```python
from build123d import *

# Parameters (mm, degrees)
BOSS_EXTRUDE1_DEPTH          = 4
SKETCH2_W                    = 4
SKETCH2_H                    = 32
BOSS_EXTRUDE2_DEPTH          = 72
CUT_EXTRUDE1_DEPTH           = 109.664621658
SKETCH4_W                    = 12.6
SKETCH4_H                    = 4
SKETCH4_W_2                  = 12.599860781
BOSS_EXTRUDE3_DEPTH          = 4
SKETCH5_R                    = 1
CUT_EXTRUDE2_DEPTH           = 4
CUT_EXTRUDE2_DRAFT           = -1
CUT_EXTRUDE2_PROFILE_2_DEPTH = 4
CUT_EXTRUDE2_PROFILE_2_DRAFT = -1
CUT_EXTRUDE4_DEPTH           = 102.980390272
BOSS_EXTRUDE6_DEPTH          = 32
BOSS_EXTRUDE7_DEPTH          = 2
SKETCH14_R                   = 18
SKETCH14_R_2                 = 16
BOSS_EXTRUDE8_DEPTH          = 4
SKETCH15_R                   = 2
CUT_EXTRUDE5_DEPTH           = 4
SKETCH16_R                   = 4
SKETCH16_R_2                 = 2
CUT_EXTRUDE6_DEPTH           = 2
SKETCH17_W                   = 5
SKETCH17_H                   = 10
CUT_EXTRUDE7_DEPTH           = 10
BOSS_EXTRUDE9_DEPTH          = 2
MIRROR6_COPY_1_DEPTH         = 2
FILLET1_R                    = 10
FILLET2_R                    = 10


with BuildPart() as part:
    # Sketch1 → Boss-Extrude1 (new body)
    with BuildSketch(Plane(origin=(0, 0, 0), x_dir=(1, 0, 0), z_dir=(0, 1, 0))):
        with BuildLine():
            Line((0, 16), (60, 16))
            Line((60, 16), (60, -16))
            Line((60, -16), (0, -16))
            ThreePointArc((0, -16), (-16, 0), (0, 16))
        make_face()
    boss_extrude1 = extrude(amount=BOSS_EXTRUDE1_DEPTH)

    # Sketch2 → Boss-Extrude2 (add)
    with BuildSketch(Plane(origin=(0, 4, 0), x_dir=(1, 0, 0), z_dir=(0, 1, 0))):
        with Locations((58, 0)):
            Rectangle(SKETCH2_W, SKETCH2_H)
    extrude(amount=BOSS_EXTRUDE2_DEPTH)

    # Mirror1: Boss-Extrude1 across plane
    add(boss_extrude1.mirror(Plane(origin=(0, 38, 0), x_dir=(0, 0, 1), z_dir=(0, -1, 0))))

    # Sketch3 → Cut-Extrude1 (cut, through all)
    with BuildSketch(Plane(origin=(60, 0, 0), x_dir=(0, 0, -1), z_dir=(1, 0, 0))):
        with BuildLine():
            ThreePointArc((-2.594812436, 43.59757706), (0, 31.830241454), (2.594812436, 43.59757706))
            ThreePointArc((2.594812436, 43.59757706), (0, 46.625832401), (-2.594812436, 43.59757706))
        make_face()
    extrude(amount=-CUT_EXTRUDE1_DEPTH, mode=Mode.SUBTRACT)

    # Sketch4 → Boss-Extrude3 (add)
    with BuildSketch(Plane.ZY.offset(-56)):
        with Locations((0, 57.55)):
            Rectangle(SKETCH4_W, SKETCH4_H)
        with Locations((8.8752e-05, 29.45)):
            Rectangle(SKETCH4_W_2, SKETCH4_H)
    extrude(amount=BOSS_EXTRUDE3_DEPTH)


with BuildPart() as cut_extrude2_tool:
    # Sketch5 → Cut-Extrude2 (with draft: the straight prism first)
    with BuildSketch(Plane.ZY.offset(-52)):
        with Locations((0, 57.275)):
            Circle(SKETCH5_R)
    extrude(amount=-CUT_EXTRUDE2_DEPTH)
    # Cut-Extrude2: the draft: its side faces are tilted about the plane it starts from
    cut_extrude2_sides = [cut_extrude2_tool.faces().sort_by_distance(p)[0] for p in [
        (54, 57.275, -1),
    ]]
    draft(cut_extrude2_sides, Plane.ZY.offset(-52), CUT_EXTRUDE2_DRAFT)


with BuildPart() as part_1:
    add(part.part)

    # Cut-Extrude2: cut by cut_extrude2_tool
    add(cut_extrude2_tool.part, mode=Mode.SUBTRACT)


with BuildPart() as cut_extrude2_profile_2_tool:
    # Sketch5 → Cut-Extrude2 profile 2 (with draft: the straight prism first)
    with BuildSketch(Plane.ZY.offset(-52)):
        with Locations((0.01512814, 29.732868428)):
            Circle(SKETCH5_R)
    extrude(amount=-CUT_EXTRUDE2_PROFILE_2_DEPTH)
    # Cut-Extrude2 profile 2: the draft: its side faces are tilted about the plane it starts from
    cut_extrude2_profile_2_sides = [cut_extrude2_profile_2_tool.faces().sort_by_distance(p)[0] for p in [
        (54, 29.732868428, -0.98487186),
    ]]
    draft(cut_extrude2_profile_2_sides, Plane.ZY.offset(-52), CUT_EXTRUDE2_PROFILE_2_DRAFT)


with BuildPart() as part_2:
    add(part_1.part)

    # Cut-Extrude2 profile 2: cut by cut_extrude2_profile_2_tool
    add(cut_extrude2_profile_2_tool.part, mode=Mode.SUBTRACT)

    # Sketch11 → Cut-Extrude4 (cut, through all)
    with BuildSketch(Plane.XY.offset(16)):
        Polygon((56, 59.55), (30, 72), (30, 76), (60, 76), (60, 59.55), align=None)
        Polygon((60, 0), (60, 14.79), (56, 14.79), (30, 4), (30, 0), align=None)
    extrude(amount=-CUT_EXTRUDE4_DEPTH, mode=Mode.SUBTRACT)


with BuildPart() as cut_extrude4_piece_1:
    # of the separate pieces the step leaves, piece 1, a body of its own (cut_extrude4_pieces)
    add(part_2.part.solids().sort_by_distance((60, 59.55, -16))[0])



with BuildPart() as cut_extrude4_piece_2:
    # of the separate pieces the step leaves, piece 2, a body of its own (cut_extrude4_pieces)
    add(part_2.part.solids().sort_by_distance((0, 0, -16))[0])


with BuildPart() as cut_extrude4_piece_3:
    # of the separate pieces the step leaves, piece 3, a body of its own (cut_extrude4_pieces)
    add(part_2.part.solids().sort_by_distance((0, 76, -16))[0])


with BuildPart() as cut_extrude4_piece_1_1:
    add(cut_extrude4_piece_1.part)

    add(cut_extrude4_piece_2.part)  # Boss-Extrude6 merges Cut-Extrude4 piece 2

    add(cut_extrude4_piece_3.part)  # Boss-Extrude6 merges Cut-Extrude4 piece 3
    # Sketch12 → Boss-Extrude6 (add, through all)
    with BuildSketch(Plane.XY.offset(16)):
        Polygon((30, 72), (56, 59.55), (60, 59.55), (60, 62.55), (30, 76), align=None)
        Polygon((30, 4), (56, 14.79), (60, 14.79), (60, 11.79), (30, 0), align=None)
    extrude(amount=-BOSS_EXTRUDE6_DEPTH)

    # Sketch13 → Boss-Extrude7 (add)
    with BuildSketch(Plane.XY.offset(16)):
        Polygon((30, 76), (30, 0), (60, 11.79), (60, 62.55), align=None)
    boss_extrude7 = extrude(amount=-BOSS_EXTRUDE7_DEPTH)

    # Mirror2: Boss-Extrude7 across plane
    add(boss_extrude7.mirror(Plane.XY))

    # Sketch14 → Boss-Extrude8 (add)
    with BuildSketch(Plane(origin=(0, 76, 0), x_dir=(1, 0, 0), z_dir=(0, 1, 0))):
        Circle(SKETCH14_R)
        Circle(SKETCH14_R_2, mode=Mode.SUBTRACT)
    boss_extrude8 = extrude(amount=-BOSS_EXTRUDE8_DEPTH)

    # Sketch15 → Cut-Extrude5 (cut)
    with BuildSketch(Plane(origin=(0, 76, 0), x_dir=(1, 0, 0), z_dir=(0, 1, 0))):
        with Locations(Location((-13.5, 0, 0), (0, 0, 270))):
            Circle(SKETCH15_R)
        with Locations(Location((-4.171729424, 12.83926297, 0), (0, 0, 270))):
            Circle(SKETCH15_R)
        with Locations(Location((10.921729424, 7.935100906, 0), (0, 0, 270))):
            Circle(SKETCH15_R)
        with Locations(Location((10.921729424, -7.935100906, 0), (0, 0, 270))):
            Circle(SKETCH15_R)
        with Locations(Location((-4.171729424, -12.83926297, 0), (0, 0, 270))):
            Circle(SKETCH15_R)
    cut_extrude5 = extrude(amount=-CUT_EXTRUDE5_DEPTH, mode=Mode.SUBTRACT)

    # Mirror3: Boss-Extrude8, Cut-Extrude5 across plane
    add(boss_extrude8.mirror(Plane(origin=(0, 38, 0), x_dir=(0, 0, 1), z_dir=(0, -1, 0))))
    add(cut_extrude5.mirror(Plane(origin=(0, 38, 0), x_dir=(0, 0, 1), z_dir=(0, -1, 0))), mode=Mode.SUBTRACT)

    # Sketch16 → Cut-Extrude6 (cut)
    # profile 1 of 5: a face of its own
    with BuildSketch(Plane.XZ):
        with Locations(Location((-4.171729424, 12.83926297, 0), (0, 0, 270))):
            Circle(SKETCH16_R)
        with Locations(Location((-4.171729424, 12.83926297, 0), (0, 0, 270))):
            Circle(SKETCH16_R_2, mode=Mode.SUBTRACT)
    # profile 2 of 5: a face of its own
    with BuildSketch(Plane.XZ):
        with Locations(Location((10.921729424, 7.935100906, 0), (0, 0, 270))):
            Circle(SKETCH16_R)
        with Locations(Location((10.921729424, 7.935100906, 0), (0, 0, 270))):
            Circle(SKETCH16_R_2, mode=Mode.SUBTRACT)
    # profile 3 of 5: a face of its own
    with BuildSketch(Plane.XZ):
        with Locations(Location((10.921729424, -7.935100906, 0), (0, 0, 270))):
            Circle(SKETCH16_R)
        with Locations(Location((10.921729424, -7.935100906, 0), (0, 0, 270))):
            Circle(SKETCH16_R_2, mode=Mode.SUBTRACT)
    # profile 4 of 5: a face of its own
    with BuildSketch(Plane.XZ):
        with Locations(Location((-4.171729424, -12.83926297, 0), (0, 0, 270))):
            Circle(SKETCH16_R)
        with Locations(Location((-4.171729424, -12.83926297, 0), (0, 0, 270))):
            Circle(SKETCH16_R_2, mode=Mode.SUBTRACT)
    # profile 5 of 5: a face of its own
    with BuildSketch(Plane.XZ):
        with Locations(Location((-13.5, 0, 0), (0, 0, 270))):
            Circle(SKETCH16_R)
        with Locations(Location((-13.5, 0, 0), (0, 0, 270))):
            Circle(SKETCH16_R_2, mode=Mode.SUBTRACT)
    cut_extrude6 = extrude(amount=-CUT_EXTRUDE6_DEPTH, mode=Mode.SUBTRACT)

    # Mirror4: Cut-Extrude6 across plane
    add(cut_extrude6.mirror(Plane(origin=(0, 38, 0), x_dir=(0, 0, 1), z_dir=(0, -1, 0))), mode=Mode.SUBTRACT)

    # Sketch17 → Cut-Extrude7 (cut)
    with BuildSketch(Plane(origin=(0, 0, -16), x_dir=(-1, 0, 0), z_dir=(0, 0, -1))):
        with Locations((-45, 38)):
            Rectangle(SKETCH17_W, SKETCH17_H)
    extrude(amount=-CUT_EXTRUDE7_DEPTH, mode=Mode.SUBTRACT)

    # Sketch18 → Boss-Extrude9 (add)
    with BuildSketch(Plane(origin=(0, 0, -16), x_dir=(-1, 0, 0), z_dir=(0, 0, -1))):
        Polygon((-30, 11), (-27, 8), (-26, 7), (-23, 4), (-30, 4), align=None)
    boss_extrude9 = extrude(amount=-BOSS_EXTRUDE9_DEPTH)

    # Mirror5: Boss-Extrude9 across plane
    add(boss_extrude9.mirror(Plane.XY))

    # Mirror6: Boss-Extrude9 across plane
    add(boss_extrude9.mirror(Plane(origin=(0, 38, 0), x_dir=(0, 0, 1), z_dir=(0, -1, 0))))

    # Mirror6 copy 1 sketch → Mirror6 copy 1 (add)
    with BuildSketch(Plane(origin=(0, 76, 16), x_dir=(-1, 0, 0), z_dir=(0, 0, 1))):
        Polygon((-30, 11), (-27, 8), (-26, 7), (-23, 4), (-30, 4), align=None)
    extrude(amount=-MIRROR6_COPY_1_DEPTH)

    # Fillet1
    fillet1_edges = [cut_extrude4_piece_1_1.edges().sort_by_distance(p)[0] for p in [
        (30, 72, 0),
    ]]
    fillet(fillet1_edges, radius=FILLET1_R)

    # Fillet2
    fillet2_edges = [cut_extrude4_piece_1_1.edges().sort_by_distance(p)[0] for p in [
        (30, 4, 0),
    ]]
    fillet(fillet2_edges, radius=FILLET2_R)


solid = cut_extrude4_piece_1_1.part
```
Check sheet for the modelled part. Datum: model origin and axes. Units: mm. A direction names the side the tool comes from. Round coordinates to 2 decimals unless told otherwise and drop trailing zeros. Loops run counter-clockwise (first coordinate to the right, second up) from the corner with the lowest first, then second, coordinate; pieces in that order, holes last. Notation, with made-up numbers: M -8,-22.75 L 29,-22.75 A27 cw 29,0.25 Z; hole C -39,-13.75 d3. An arc over 180 degrees is marked long. Answer as a JSON object with one key per item and string values.
1. Section check D-D (y = 20). Record the boundary of the cut face in (x, z), plus the area to 3 significant figures.
Reply:
{"outline": "M 30,-16 L 60,-16 L 60,16 L 30,16 L 30,14 L 56,14 L 56,-14 L 30,-14 Z", "area": "232 mm²"}
2. Access from +Z, -Z, +X, -X, +Y, -Y to the whole of each face (thin tool, end or side, straight path). Record for faces 1 (the flat face through (45, 33, -15)), 2 (the flat face through (26, 69, -15)), 3 (the cylindrical face through (13.63, 75.01, 10.88)).
Reply:
{"face 1": "-Z", "face 2": "+Z, -Z, -X", "face 3": "+Y"}
3. Section check C-C (x = 1). Record the boundary of the cut face in (y, z), plus the area to 3 significant figures.
Reply:
{"outline": "M 0,-17.97 L 4,-17.97 L 4,17.97 L 0,17.97 Z; M 72,-17.97 L 76,-17.97 L 76,17.97 L 72,17.97 Z", "area": "288 mm²"}
4. Section check B-B (z = 13). State how many separate pieces and enclosed holes the cut face has, plus the area to 3 significant figures.
Reply:
{"separate pieces": "3", "enclosed holes": "0", "area": "728 mm²"}
5. Mould release check, pull along X, two halves, no side actions. Record for faces 4 (the flat face through (5, 4, 0)), 5 (the flat face through (30, 38, 15)), 6 (the flat face through (13, 2, -9)): pulls with the +X half, pulls with the -X half, needs draft (parallel to the pull), parting line crosses it, or undercut.
Reply:
{"face 4": "needs draft", "face 5": "pulls with the -X half", "face 6": "undercut"}
6. Gauge pin test, flat ends, axial feed: P1, Ø12, axis at y = 11.5, z = -2.5, coming from the -X side; P2, Ø4, axis at y = 61, z = -6.5, coming from the -X side; P3, Ø7, axis at x = -4.17, z = -12.84, coming from the +Y side. Record the tip position at first contact, or that the pin passes through.
Reply:
{"P1": "stops at x = 33.61", "P2": "stops at x = 48.8", "P3": "stops at y = 74"}
7. Scan lines: line 1 (Y direction, x = 17, z = 9); line 2 (Z direction, x = 41, y = 44); line 3 (Y direction, x = 7, z = -8). Record each from-to range of solid material in increasing order.
Reply:
{"line 1": "y = 0 to 4, 72 to 76", "line 2": "z = -16 to -14, 14 to 16", "line 3": "y = 2 to 4, 72 to 74"}
8. Section check A-A (y = 38). Record the boundary of the cut face in (x, z), plus the area to 3 significant figures.
Reply:
{"outline": "M 30,-16 L 42.5,-16 L 42.5,-14 L 30,-14 Z; M 30,14 L 56,14 L 56,6.17 L 60,6.17 L 60,16 L 30,16 Z; M 47.5,-16 L 60,-16 L 60,-6.17 L 56,-6.17 L 56,-14 L 47.5,-14 Z", "area": "173 mm²"}
